Verification items for the finished model (mm, model axes). A direction names the side the tool comes from. Coordinates: 2 decimals unless noted, no trailing zeros. Order: outer loops, then holes, each group sorted by start corner. A loop starts at its lowest first (then second) coordinate and runs counter-clockwise, first axis right, second up. Notation, with made-up numbers: M 63.5,-22.75 L 72.5,-22.75 A13 cw 72.5,-14.75 Z; hole C -22.5,-25 d5. An arc over 180 degrees is marked long. Write item = value, one per line.
```python
from build123d import *

# Parameters (mm, degrees)
F1_DEPTH = 63.5
F3_DEPTH = 72.136
F4_DEPTH = 31.75


with BuildPart() as f1:
    # F0 (on Front) → F1 (new body)
    with BuildSketch(Plane.XZ):
        Polygon((65.964764, 38.1), (-61.035236, 38.1), (-61.035236, 0), (2.464764, 0), (65.979816, 0), (65.964764, 19.05), align=None)
    extrude(amount=F1_DEPTH)

    # F2 (on Front) → F3 (cut)
    with BuildSketch(Plane.XZ):
        Polygon((2.483717, 0), (65.983717, 0), (65.983717, 19.056977), (2.487009, 19.056977), align=None)
    extrude(amount=F3_DEPTH, mode=Mode.SUBTRACT)

    # F2 (on Front) → F4 (join)
    with BuildSketch(Plane.XZ):
        Polygon((2.483717, 0), (65.983717, 0), (65.983717, 19.056977), (2.487009, 19.056977), align=None)
    extrude(amount=F4_DEPTH)


solid = f1.part
```
Item 1: Scan lines: L1, parallel to Y at x = 44.5, z = 8; L2, parallel to X at y = -52, z = 22; L3, parallel to X at y = -59, z = 16. Record each from-to range of solid material in increasing order. Write a range as from..to.
Report:
L1 = -31.75..0
L2 = -61.04..65.96
L3 = -61.04..2.49
Item 2: Gauge pin test, flat ends, axial feed: pin 1 (5.5 mm diameter, centred on x = 37.5, z = 12, fed in from -Y); pin 2 (15 mm diameter, centred on y = -41, z = 8.5, fed in from +X); pin 3 (4 mm diameter, centred on x = -3.5, y = -7, fed in from -Z); pin 4 (1.5 mm diameter, centred on y = -50, z = 29, fed in from +X). Record the tip position at first contact, or that the pin passes through.
Report:
pin_1 = -31.75
pin_2 = 2.49
pin_3 = 0
pin_4 = 65.96
Item 3: Sectioned sample at B-B, the plane y = -59. Enter the section's corners in (x, z), then the cut area to 3 significant figures.
Report:
outline = M -61.04,0 L 2.48,0 L 2.49,19.06 L 65.96,19.06 L 65.96,38.1 L -61.04,38.1 Z
area = 3,630 mm^2
Item 4: Sectioned sample at A-A, the plane x = 10. Enter the section's corners in (y, z), then the cut area to 3 significant figures.
Report:
outline = M -63.5,19.06 L -31.75,19.06 L -31.75,0 L 0,0 L 0,38.1 L -63.5,38.1 Z
area = 1,810 mm^2
Item 5: Tool access check on faces 1 (the flat face through (35, -47, 19.057)), 2 (the flat face through (2, 0, 19)). Record the directions out of +Z, -Z, +X, -X, +Y, -Y that give a thin tool (end or side, any length) a straight path to the whole face; none if there is none.
Report:
face_1 = -Z, +X, -Y
face_2 = +Z, -Z, +X, -X, +Y
